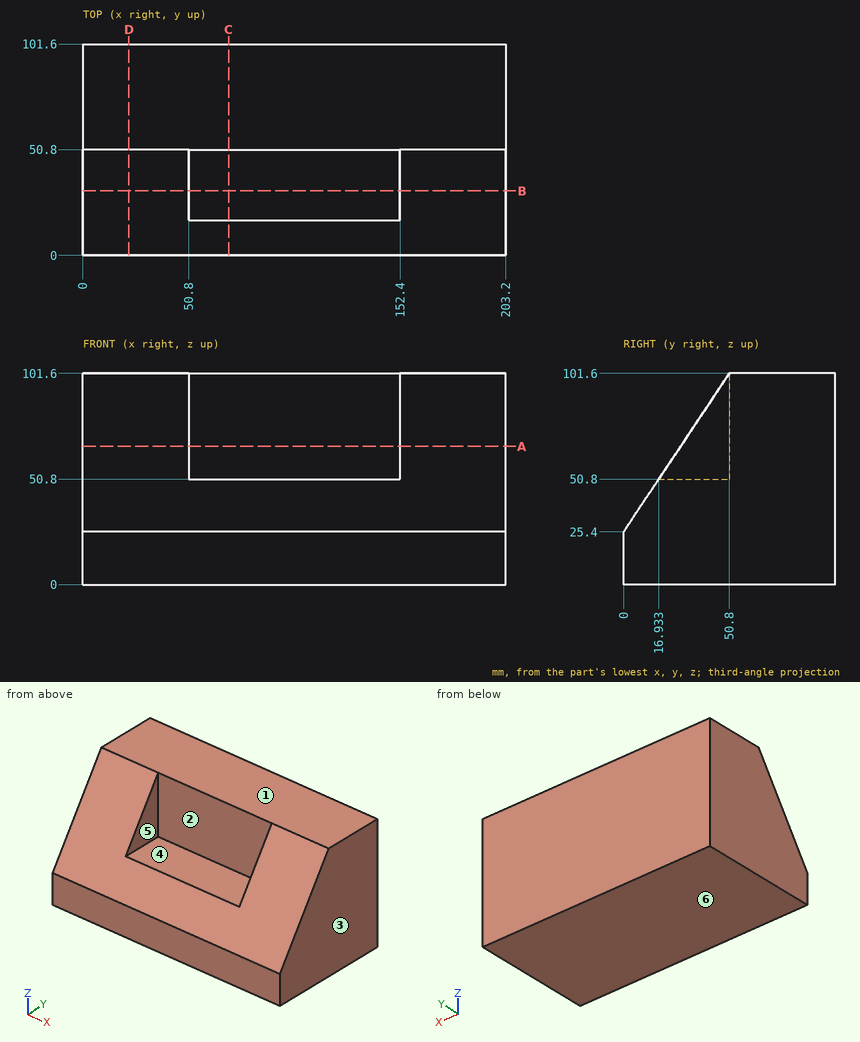
Could you check a few things on this drawing? It's one solid part, dimensions in mm from its lowest x, y, z. A direction names the side the tool comes from. Coordinates: 2 decimals unless noted, no trailing zeros. Order: outer loops, then holes, each group sorted by start corner. A loop starts at its lowest first (then second) coordinate and runs counter-clockwise, first axis right, second up. Notation, with made-up numbers: M 2.5,85 L 40.5,85 A38 cw 40.5,124 Z; hole C 78,4 d2. An arc over 180 degrees is marked long. Answer as a JSON object with one key per item and string values. Group by question number.
(1) Suppose I cut it at D-D, the plane x = 22. Please give me the cut outline in (y, z).
(2) Which directions (+Z, -Z, +X, -X, +Y, -Y) give clear straight access to the entire face, cutting with the end or side of a thin tool? Please do the marked faces 5 and 6.
(3) I need wall thicknesses on probe 1 along X at (y, z) = (50, 77); probe 2 along Y at (x, z) = (74, 92.5); probe 3 along Z at (x, y) = (87, 22). Which ranges of each line are inside material? Lowest first, please.
(4) For pin 1 (6 mm diameter, centred on x = 132, y = 26.5, fed in from +Z); pin 2 (8 mm diameter, centred on x = 136, y = 63, fed in from -Z), each with a flat end and sliding along its axis, tell me the tip position at first contact or that it passes through.
(5) Suppose I cut it at C-C, the plane x = 70. Please give me the cut outline in (y, z).
(6) Suppose I cut it at B-B, the plane y = 31. Please give me the cut outline in (x, z), then the cut area to 3 significant figures.
(7) If we mould it in two halves opening along X, with no side actions, what happens to the marked faces 1, 2, 3 and 4? For each: released by +X, released by -X, zero draft, split by the parting line, or undercut.
(8) Suppose I cut it at A-A, the plane z = 66.5. Please give me the cut outline in (x, y), then the cut area to 3 significant figures.
Values found:
{
 "1": {"outline": "M 0,0 L 101.6,0 L 101.6,101.6 L 50.8,101.6 L 0,25.4 Z"},
 "2": {"face 5": "+Z, -Y", "face 6": "-Z, +X, -X, +Y, -Y"},
 "3": {"probe 1": "x = 0 to 50.8, 152.4 to 203.2", "probe 2": "y = 50.8 to 101.6", "probe 3": "z = 0 to 50.8"},
 "4": {"pin 1": "stops at z = 50.8", "pin 2": "stops at z = 0"},
 "5": {"outline": "M 0,0 L 101.6,0 L 101.6,101.6 L 50.8,101.6 L 50.8,50.8 L 16.93,50.8 L 0,25.4 Z"},
 "6": {"outline": "M 0,0 L 203.2,0 L 203.2,71.9 L 152.4,71.9 L 152.4,50.8 L 50.8,50.8 L 50.8,71.9 L 0,71.9 Z", "area": "12,500 mm^2"},
 "7": {"face 1": "zero draft", "face 2": "undercut", "face 3": "released by +X", "face 4": "undercut"},
 "8": {"outline": "M 0,27.4 L 50.8,27.4 L 50.8,50.8 L 152.4,50.8 L 152.4,27.4 L 203.2,27.4 L 203.2,101.6 L 0,101.6 Z", "area": "12,700 mm^2"}
}
